Autodesk Inventor part; units mm, degrees
ref_plane "YZ Plane" through (0, 0, 0) normal (1, 0, 0) x (0, 1, 0)
ref_plane "XZ Plane" through (0, 0, 0) normal (0, 1, 0) x (-1, 0, 0)
ref_plane "XY Plane" through (0, 0, 0) normal (0, 0, 1) x (1, 0, 0)
sketch "Эскиз1" plane through (0, 0, 0) normal (0, 1, 0) x (-1, 0, 0)
  line L0 (6.5, -2.54) -> (-6.5, -2.54)
  line L1 (-6.5, -2.54) -> (-6.5, 2.54)
  line L2 (-6.5, 2.54) -> (6.5, 2.54)
  line L3 (6.5, 2.54) -> (6.5, -2.54)
  line L4 (0, -3.556) -> (0, 3.556)
  line L5 (9.1, 0) -> (-9.1, 0)
  point P0 (0, 0)
  dimension "d0" = 13
  dimension "d1" = 5.08
extrude "Выдавливание1" add sketch "Эскиз1" along normal blind 4.4
sketch "Эскиз2" plane through (0, 4.4, 0) normal (0, 1, 0) x (1, 0, 0)
  line L0 (-5.48, 1.67) -> (-4.68, 1.67)
  line L1 (-4.68, 1.67) -> (-4.68, 0.87)
  line L2 (-4.68, 0.87) -> (-5.48, 0.87)
  line L3 (-5.48, 0.87) -> (-5.48, 1.67)
  line L4 (-2.94, 1.67) -> (-2.14, 1.67)
  line L5 (-2.14, 1.67) -> (-2.14, 0.87)
  line L6 (-2.14, 0.87) -> (-2.94, 0.87)
  line L7 (-2.94, 0.87) -> (-2.94, 1.67)
  line L8 (-0.4, 1.67) -> (0.4, 1.67)
  line L9 (0.4, 1.67) -> (0.4, 0.87)
  line L10 (0.4, 0.87) -> (-0.4, 0.87)
  line L11 (-0.4, 0.87) -> (-0.4, 1.67)
  line L12 (2.14, 1.67) -> (2.94, 1.67)
  line L13 (2.94, 1.67) -> (2.94, 0.87)
  line L14 (2.94, 0.87) -> (2.14, 0.87)
  line L15 (2.14, 0.87) -> (2.14, 1.67)
  line L16 (4.68, 1.67) -> (5.48, 1.67)
  line L17 (5.48, 1.67) -> (5.48, 0.87)
  line L18 (5.48, 0.87) -> (4.68, 0.87)
  line L19 (4.68, 0.87) -> (4.68, 1.67)
  line L20 (-5.48, -0.87) -> (-4.68, -0.87)
  line L21 (-4.68, -0.87) -> (-4.68, -1.67)
  line L22 (-4.68, -1.67) -> (-5.48, -1.67)
  line L23 (-5.48, -1.67) -> (-5.48, -0.87)
  line L24 (-2.94, -0.87) -> (-2.14, -0.87)
  line L25 (-2.14, -0.87) -> (-2.14, -1.67)
  line L26 (-2.14, -1.67) -> (-2.94, -1.67)
  line L27 (-2.94, -1.67) -> (-2.94, -0.87)
  line L28 (-0.4, -0.87) -> (0.4, -0.87)
  line L29 (0.4, -0.87) -> (0.4, -1.67)
  line L30 (0.4, -1.67) -> (-0.4, -1.67)
  line L31 (-0.4, -1.67) -> (-0.4, -0.87)
  line L32 (2.14, -0.87) -> (2.94, -0.87)
  line L33 (2.94, -0.87) -> (2.94, -1.67)
  line L34 (2.94, -1.67) -> (2.14, -1.67)
  line L35 (2.14, -1.67) -> (2.14, -0.87)
  line L36 (4.68, -0.87) -> (5.48, -0.87)
  line L37 (5.48, -0.87) -> (5.48, -1.67)
  line L38 (5.48, -1.67) -> (4.68, -1.67)
  line L39 (4.68, -1.67) -> (4.68, -0.87)
  line L40 (0, 3.556) -> (0, -3.556)
  line L41 (-9.1, 0) -> (9.1, 0)
  point P0 (0, 0)
  dimension "d4" = 0.8
  dimension "d5" = 0.8
  dimension "d8" = 2.54
  dimension "d11" = 2.54
extrude "Выдавливание2" cut sketch "Эскиз2" against normal blind 4
sketch "Эскиз3" plane through (0, 0, 0) normal (0, -1, 0) x (1, 0, 0)
  line L0 (0, -3.556) -> (0, 3.556)
  line L1 (-9.1, 0) -> (9.1, 0)
  line L2 (-5.48, 1.42) -> (-4.68, 1.42)
  line L3 (-4.68, 1.42) -> (-4.68, 1.12)
  line L4 (-4.68, 1.12) -> (-5.48, 1.12)
  line L5 (-5.48, 1.12) -> (-5.48, 1.42)
  line L6 (-2.94, 1.42) -> (-2.14, 1.42)
  line L7 (-2.14, 1.42) -> (-2.14, 1.12)
  line L8 (-2.14, 1.12) -> (-2.94, 1.12)
  line L9 (-2.94, 1.12) -> (-2.94, 1.42)
  line L10 (-0.4, 1.42) -> (0.4, 1.42)
  line L11 (0.4, 1.42) -> (0.4, 1.12)
  line L12 (0.4, 1.12) -> (-0.4, 1.12)
  line L13 (-0.4, 1.12) -> (-0.4, 1.42)
  line L14 (2.14, 1.42) -> (2.94, 1.42)
  line L15 (2.94, 1.42) -> (2.94, 1.12)
  line L16 (2.94, 1.12) -> (2.14, 1.12)
  line L17 (2.14, 1.12) -> (2.14, 1.42)
  line L18 (4.68, 1.42) -> (5.48, 1.42)
  line L19 (5.48, 1.42) -> (5.48, 1.12)
  line L20 (5.48, 1.12) -> (4.68, 1.12)
  line L21 (4.68, 1.12) -> (4.68, 1.42)
  line L22 (-5.48, -1.12) -> (-4.68, -1.12)
  line L23 (-4.68, -1.12) -> (-4.68, -1.42)
  line L24 (-4.68, -1.42) -> (-5.48, -1.42)
  line L25 (-5.48, -1.42) -> (-5.48, -1.12)
  line L26 (-2.94, -1.12) -> (-2.14, -1.12)
  line L27 (-2.14, -1.12) -> (-2.14, -1.42)
  line L28 (-2.14, -1.42) -> (-2.94, -1.42)
  line L29 (-2.94, -1.42) -> (-2.94, -1.12)
  line L30 (-0.4, -1.12) -> (0.4, -1.12)
  line L31 (0.4, -1.12) -> (0.4, -1.42)
  line L32 (0.4, -1.42) -> (-0.4, -1.42)
  line L33 (-0.4, -1.42) -> (-0.4, -1.12)
  line L34 (2.14, -1.12) -> (2.94, -1.12)
  line L35 (2.94, -1.12) -> (2.94, -1.42)
  line L36 (2.94, -1.42) -> (2.14, -1.42)
  line L37 (2.14, -1.42) -> (2.14, -1.12)
  line L38 (4.68, -1.12) -> (5.48, -1.12)
  line L39 (5.48, -1.12) -> (5.48, -1.42)
  line L40 (5.48, -1.42) -> (4.68, -1.42)
  line L41 (4.68, -1.42) -> (4.68, -1.12)
  point P0 (0, 0)
  dimension "d16" = 0.8
  dimension "d17" = 0.3
  dimension "d20" = 2.54
  dimension "d23" = 2.54
extrude "Выдавливание3" add sketch "Эскиз3" along normal blind 2
properties part number "MOLEX"
Model file for the job. Use its own axes, mm. A direction names the side the tool comes from. Round coordinates to 2 decimals unless told otherwise and drop trailing zeros. Order: outer loops, then holes, each group sorted by start corner. A loop starts at its lowest first (then second) coordinate and runs counter-clockwise, first axis right, second up. Notation, with made-up numbers: M 39,7.25 L 86,7.25 A23 ccw 86,25.25 Z; hole C -2,63 d1. An arc over 180 degrees is marked long. Write each question's results on one line, items separated by ' | '. Start each with the question number.
(1) Probe probe 1 along X at (y, z) = (2.5, -1.55); probe 2 along Z at (x, y) = (-2.25, 4); probe 3 along Z at (x, y) = (-5, -0.25). List the from-to ranges inside material, lowest first. Write a range as from..to.
(2) Drop a flat-ended pin along its axis: pin 1 (0.9 mm diameter, centred on x = 2.5, y = -1, fed in from -Z). Give the stop position or say it passes through.
(3) Saw through at A-A, the plane x = 5. Give the cut face in (y, z).
(4) Two-plate mould, pull along Z, no slides. Class faces 5 (the face through (5, -1, -1.42)), 6 (the face through (0, 4.4, 0)), 7 (the face through (-5, 2, -0.87)): pulls with the +Z half, pulls with the -Z half, needs draft (parallel to the pull), parting line crosses it, or undercut.
(5) Which spindle directions (+Z, -Z, +X, -X, +Y, -Y) get a long thin tool onto all of the face, cutting with end or side? Do faces 1 (the face through (5, -1, -1.12)), 2 (the face through (-5, 2, -1.67)), 3 (the face through (-5, -1, -1.42)), 4 (the face through (6.5, 2, 0)). Say none if no direction does.
(6) Saw through at B-B, the plane y = 4.25. State how many separate pieces and enclosed holes the cut face has, then the cut area to 3 significant figures.
(7) Saw through at D-D, the plane z = 0.6. Give the cut face in (x, y), then the cut area to 3 significant figures.
Established:
1) probe 1: x = -6.5..-5.48, -4.68..-2.94, -2.14..-0.4, 0.4..2.14, 2.94..4.68, 5.48..6.5 | probe 2: z = -2.54..-1.67, -0.87..0.87, 1.67..2.54 | probe 3: z = -1.42..-1.12, 1.12..1.42
2) pin 1: stops at z = -1.42
3) outline: M -2,-1.42 L 0,-1.42 L 0,-2.54 L 4.4,-2.54 L 4.4,-1.67 L 0.4,-1.67 L 0.4,-0.87 L 4.4,-0.87 L 4.4,0.87 L 0.4,0.87 L 0.4,1.67 L 4.4,1.67 L 4.4,2.54 L 0,2.54 L 0,1.42 L -2,1.42 L -2,1.12 L 0,1.12 L 0,-1.12 L -2,-1.12 Z
4) face 5: pulls with the -Z half | face 6: needs draft | face 7: undercut
5) face 1: +X, -X, -Y | face 2: +Y | face 3: -Z, +X, -X, -Y | face 4: +Z, -Z, +X, +Y, -Y
6) separate pieces: 1 | enclosed holes: 10 | area: 59.6 mm^2
7) outline: M -6.5,0 L 6.5,0 L 6.5,4.4 L -6.5,4.4 Z | area: 57.2 mm^2
